Read the model definition and answer for the solid it produces. Units are mm, in the model's axes. Face numbers are marked on the shaded views. A direction names the side the tool comes from. Give positions to 0.01 mm unless a question says otherwise; leave off trailing zeros. Write each loop counter-clockwise with the first axis right and the second up, starting at its lowest first coordinate (ties: lowest second). Pieces come first, ordered by that corner, then holes. Notation, with made-up numbers: M 63.5,72 L 101.5,72 A27 cw 101.5,97 Z; hole C 80.25,31.25 d4. An arc over 180 degrees is marked long. Put each result on its own line as item: value.
from build123d import *

# Parameters (mm, degrees)
SKETCH1_R                 = 3.6
SKETCH1_R_2               = 1.6
BOSS_EXTRUDE1_DEPTH       = 5
SKETCH2_W                 = 62.8
SKETCH2_H                 = 70
BOSS_EXTRUDE2_DEPTH       = 2
F_1_0MM_DOWEL_HOLE2_D     = 2.9
F_1_0MM_DOWEL_HOLE2_DEPTH = 9.128752102
F_1_0MM_DOWEL_HOLE2_TIP   = 0.871247898
F_1_0MM_DOWEL_HOLE3_D     = 2.9
F_1_0MM_DOWEL_HOLE3_DEPTH = 9.128752102
F_1_0MM_DOWEL_HOLE3_TIP   = 0.871247898


with BuildPart() as part:
    # Sketch1 → Boss-Extrude1 (new body)
    with BuildSketch(Plane.XY):
        with Locations((-33, -19.66)):
            Circle(SKETCH1_R)
        with Locations((-33, -19.66)):
            Circle(SKETCH1_R_2, mode=Mode.SUBTRACT)
        with Locations((-33, -19.66)):
            Circle(SKETCH1_R_2)
        with Locations((-33, 8.34)):
            Circle(SKETCH1_R)
        with Locations((17.8, -23.54)):
            Circle(SKETCH1_R)
        with Locations((17.8, 23.54)):
            Circle(SKETCH1_R)
    extrude(amount=BOSS_EXTRUDE1_DEPTH)

    # Sketch2 → Boss-Extrude2 (add)
    with BuildSketch(Plane.XY.offset(5)):
        with Locations((-7.6, 0.13)):
            Rectangle(SKETCH2_W, SKETCH2_H)
    extrude(amount=BOSS_EXTRUDE2_DEPTH)

    # Ø1.0mm Dowel Hole2
    with Locations(Plane(origin=(8.8, -32.37, 7), x_dir=(1, 0, 0), z_dir=(0, 0, 1))):
        with Locations((0, 0), (-39.8, 0), (-39.8, 65), (0, 65)):
            Hole(F_1_0MM_DOWEL_HOLE2_D / 2, depth=F_1_0MM_DOWEL_HOLE2_DEPTH)
            with Locations((0, 0, -(F_1_0MM_DOWEL_HOLE2_DEPTH + F_1_0MM_DOWEL_HOLE2_TIP / 2))):  # 118° drill point
                Cone(0, F_1_0MM_DOWEL_HOLE2_D / 2, F_1_0MM_DOWEL_HOLE2_TIP, mode=Mode.SUBTRACT)

    # Ø1.0mm Dowel Hole3
    with Locations(Plane(origin=(17.8, 23.54, 0), x_dir=(-1, 0, 0), z_dir=(0, 0, -1))):
        with Locations((0, 0), (50.8, -15.2), (50.8, -43.2), (0, -47.08)):
            Hole(F_1_0MM_DOWEL_HOLE3_D / 2, depth=F_1_0MM_DOWEL_HOLE3_DEPTH)
            with Locations((0, 0, -(F_1_0MM_DOWEL_HOLE3_DEPTH + F_1_0MM_DOWEL_HOLE3_TIP / 2))):  # 118° drill point
                Cone(0, F_1_0MM_DOWEL_HOLE3_D / 2, F_1_0MM_DOWEL_HOLE3_TIP, mode=Mode.SUBTRACT)


solid = part.part
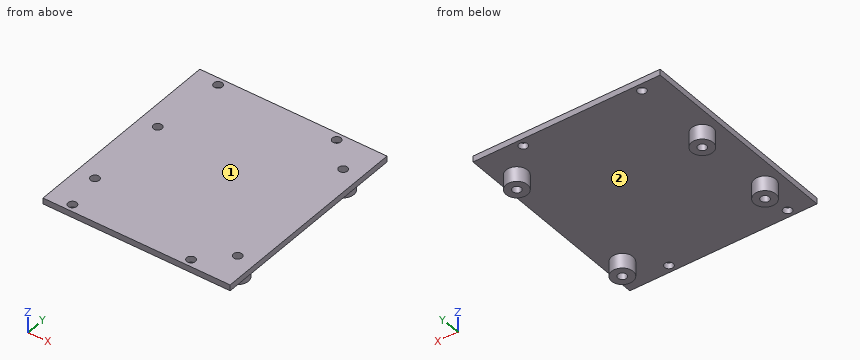
(1) Which of the six approach directions +Z, -Z, +X, -X, +Y, -Y give full straight-line access (tool end or side, diameter ignored) to the marked faces 1 and 2?
Result:
face 1: +Z, +X, -X, +Y, -Y
face 2: -Z
(2) Given pin 1 Ø4.5 at (x, y) = (-33, -19.66) entering from -Z; pin 2 Ø5 at (x, y) = (3, 23) entering from -Z; pin 3 Ø2 at (x, z) = (-23.5, 2.5) entering from +Y, each flat-ended and moving along its own axis, determine where each tip first touches the part or whether it passes through.
Result:
pin 1: stops at z = 0
pin 2: stops at z = 5
pin 3: passes through
(3) Section B-B on y = 23.54 is taken. Determine the outline of the cut face in (x, z), and give its area (3 significant figures).
Result:
outline: M -39,5 L 14.2,5 L 14.2,0 L 16.35,0 L 16.35,7 L -39,7 Z; M 19.25,0 L 21.4,0 L 21.4,5 L 23.8,5 L 23.8,7 L 19.25,7 Z
area: 141 mm²
(4) Section C-C on x = 17.8 is taken. Determine the outline of the cut face in (y, z), and give its area (3 significant figures).
Result:
outline: M -34.87,5 L -27.14,5 L -27.14,0 L -24.99,0 L -24.99,7 L -34.87,7 Z; M -22.09,0 L -19.94,0 L -19.94,5 L 19.94,5 L 19.94,0 L 22.09,0 L 22.09,7 L -22.09,7 Z; M 24.99,0 L 27.14,0 L 27.14,5 L 35.13,5 L 35.13,7 L 24.99,7 Z
area: 171 mm²
(5) Section A-A on z = 3 is taken. Determine the outline of the cut face in (x, y).
Result:
outline: C -33,-19.66 d7.2; C -33,8.34 d7.2; C 17.8,-23.54 d7.2; C 17.8,23.54 d7.2; hole C -33,-19.66 d2.9; hole C -33,8.34 d2.9; hole C 17.8,-23.54 d2.9; hole C 17.8,23.54 d2.9
(6) Straight lines are drawn through the part: line 1 along Y through (x, z) = (8.8, 5.5); line 2 along Z through (x, y) = (11.5, 8); line 3 along X through (y, z) = (23, 4.25). For each, find the intervals that lie inside material, in ascending order. Write a range as from..to.
Result:
line 1: y = -34.87..-33.82, -30.92..31.18, 34.08..35.13
line 2: z = 5..7
line 3: x = 14.24..16.45, 19.15..21.36
(7) Section D-D on y = 13.5 is taken. Determine the outline of the cut face in (x, z), and give its area (3 significant figures).
Result:
outline: M -39,5 L 23.8,5 L 23.8,7 L -39,7 Z
area: 126 mm²
